from build123d import *
from build123d.topology import SkipClean

# Parameters (mm, degrees)
CROQUIS1_W              = 90
CROQUIS1_H              = 90
SALIENTE_EXTRUIR1_DEPTH = 10
CROQUIS2_W              = 51
CROQUIS2_H              = 51
CORTAR_EXTRUIR1_DEPTH   = 4
CROQUIS3_W              = 45
CROQUIS3_H              = 45
CORTAR_EXTRUIR2_DEPTH   = 128.42056349
CROQUIS4_R              = 5
CORTAR_EXTRUIR3_DEPTH   = 128.671453348
REDONDEO1_R             = 5
REDONDEO2_R             = 25


with BuildPart() as part:
    # Croquis1 → Saliente-Extruir1 (new body)
    with BuildSketch(Plane(origin=(0, 0, 0), x_dir=(1, 0, 0), z_dir=(0, 1, 0))):
        with Locations((45, 45)):
            Rectangle(CROQUIS1_W, CROQUIS1_H)
    extrude(amount=SALIENTE_EXTRUIR1_DEPTH)

    # Croquis2 → Cortar-Extruir1 (cut)
    with BuildSketch(Plane(origin=(0, 10, 0), x_dir=(1, 0, 0), z_dir=(0, 1, 0))):
        with Locations((45, 45)):
            Rectangle(CROQUIS2_W, CROQUIS2_H)
    extrude(amount=-CORTAR_EXTRUIR1_DEPTH, mode=Mode.SUBTRACT)

    # Croquis3 → Cortar-Extruir2 (cut, through all)
    with BuildSketch(Plane(origin=(0, 6, 0), x_dir=(1, 0, 0), z_dir=(0, 1, 0))):
        with Locations((45, 45)):
            Rectangle(CROQUIS3_W, CROQUIS3_H)
    extrude(amount=-CORTAR_EXTRUIR2_DEPTH, mode=Mode.SUBTRACT)

    # Croquis4 → Cortar-Extruir3 (cut, through all)
    with SkipClean():  # the faces are left unmerged after this step: merging them gives an invalid solid
        with BuildSketch(Plane(origin=(0, 10, 0), x_dir=(1, 0, 0), z_dir=(0, 1, 0))):
            with Locations((19.5, 70.5)):
                Circle(CROQUIS4_R)
            with Locations((70.5, 70.5)):
                Circle(CROQUIS4_R)
            with Locations((19.5, 19.5)):
                Circle(CROQUIS4_R)
            with Locations((70.5, 19.5)):
                Circle(CROQUIS4_R)
        extrude(amount=-CORTAR_EXTRUIR3_DEPTH, mode=Mode.SUBTRACT)
    add(part.part.scale(1), mode=Mode.REPLACE)  # the faces are merged on a copy

    # Redondeo1
    redondeo1_edges = [part.edges().sort_by_distance(p)[0] for p in [
        (23.5, 3, -67.5),
        (22.5, 3, -66.5),
        (67.5, 3, -66.5),
        (66.5, 3, -67.5),
        (22.5, 3, -23.5),
        (23.5, 3, -22.5),
        (66.5, 3, -22.5),
        (67.5, 3, -23.5),
    ]]
    fillet(redondeo1_edges, radius=REDONDEO1_R)

    # Redondeo2
    redondeo2_edges = [part.edges().sort_by_distance(p)[0] for p in [
        (0, 5, -90),
        (90, 5, -90),
        (90, 5, 0),
        (0, 5, 0),
    ]]
    fillet(redondeo2_edges, radius=REDONDEO2_R)


solid = part.part
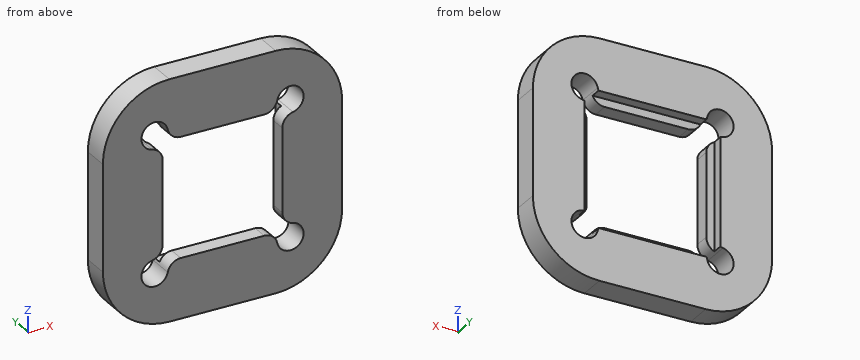
Can you work these out from the model? Positions are in its coordinate system, mm. Coordinates: 2 decimals unless noted, no trailing zeros. Write each loop counter-clockwise with the first axis right and the second up, starting at its lowest first coordinate (ties: lowest second). Pieces come first, ordered by that corner, then holes. Notation, with made-up numbers: (45, 38) -> (56, 38) arc R15 ccw to (56, 48) -> close; hole circle Ø2 at (44, 56). An arc over 180 degrees is marked (long way). Answer as CSV lines item,"result".
1) If we section it at C-C on z = -43: Please give me the cut outline in (x, y).
Check result:
outline,"(0, 0) -> (22.5, 0) -> (22.5, 6) -> (19.5, 6) -> (19.5, 10) -> (0, 10) -> close; (67.5, 0) -> (90, 0) -> (90, 10) -> (70.5, 10) -> (70.5, 6) -> (67.5, 6) -> close"
2) If we section it at A-A on x = 38.5: Please give me the cut outline in (y, z).
Check result:
outline,"(0, -90) -> (10, -90) -> (10, -70.5) -> (6, -70.5) -> (6, -67.5) -> (0, -67.5) -> close; (0, -22.5) -> (6, -22.5) -> (6, -19.5) -> (10, -19.5) -> (10, 0) -> (0, 0) -> close"
3) If we section it at D-D on y = 8.75: Please give me the cut outline in (x, z).
Check result:
outline,"(0, -65) arc R25 ccw to (25, -90) -> (65, -90) arc R25 ccw to (90, -65) -> (90, -25) arc R25 ccw to (65, 0) -> (25, 0) arc R25 ccw to (0, -25) -> close; hole (18.5, -65.6) arc R5 ccw (long way) to (24.4, -71.5) arc R5 cw to (24.72, -70.5) -> (65.28, -70.5) arc R5 cw to (65.6, -71.5) arc R5 ccw (long way) to (71.5, -65.6) arc R5 cw to (70.5, -65.28) -> (70.5, -24.72) arc R5 cw to (71.5, -24.4) arc R5 ccw (long way) to (65.6, -18.5) arc R5 cw to (65.28, -19.5) -> (24.72, -19.5) arc R5 cw to (24.4, -18.5) arc R5 ccw (long way) to (18.5, -24.4) arc R5 cw to (19.5, -24.72) -> (19.5, -65.28) arc R5 cw to start"
4) If I drill on line 1 (Z direction, x = 19.5, y = 3); line 2 (Z direction, x = 20.5, y = 0.75); line 3 (X direction, y = 6.75, z = -61), over which ranges is the centre line in solid material (lowest first)? Write a range as from..to.
Check result:
line 1,"-89.39..-75.5, -65.28..-24.72, -14.5..-0.61"
line 2,"-89.59..-75.4, -64.7..-25.3, -14.6..-0.41"
line 3,"0..19.5, 70.5..90"
5) Will these pins go through, and if not, where does the flat tip stop? P1, Ø8, axis at x = 19.5, z = -70.5, coming from the +Y side (1 decimal); P2, Ø1.5, axis at y = 5, z = -20, coming from the +X side; P3, Ø0.9, axis at x = 47.5, z = -69, coming from the +Y side; P4, Ø1.5, axis at y = 3.5, z = -22.5, coming from the +X side.
Check result:
P1,"through"
P2,"x = 89.64"
P3,"y = 6"
P4,"x = 89.94"
6) If we section it at B-B on y = 4.25: Please give me the cut outline in (x, z), then the cut area to 3 significant figures.
Check result:
outline,"(0, -65) arc R25 ccw to (25, -90) -> (65, -90) arc R25 ccw to (90, -65) -> (90, -25) arc R25 ccw to (65, 0) -> (25, 0) arc R25 ccw to (0, -25) -> close; hole (18.5, -65.6) arc R5 ccw (long way) to (24.4, -71.5) arc R5 cw to (29.3, -67.5) -> (60.7, -67.5) arc R5 cw to (65.6, -71.5) arc R5 ccw (long way) to (71.5, -65.6) arc R5 cw to (67.5, -60.7) -> (67.5, -29.3) arc R5 cw to (71.5, -24.4) arc R5 ccw (long way) to (65.6, -18.5) arc R5 cw to (60.7, -22.5) -> (29.3, -22.5) arc R5 cw to (24.4, -18.5) arc R5 ccw (long way) to (18.5, -24.4) arc R5 cw to (22.5, -29.3) -> (22.5, -60.7) arc R5 cw to start"
area,"5,180 mm²"
